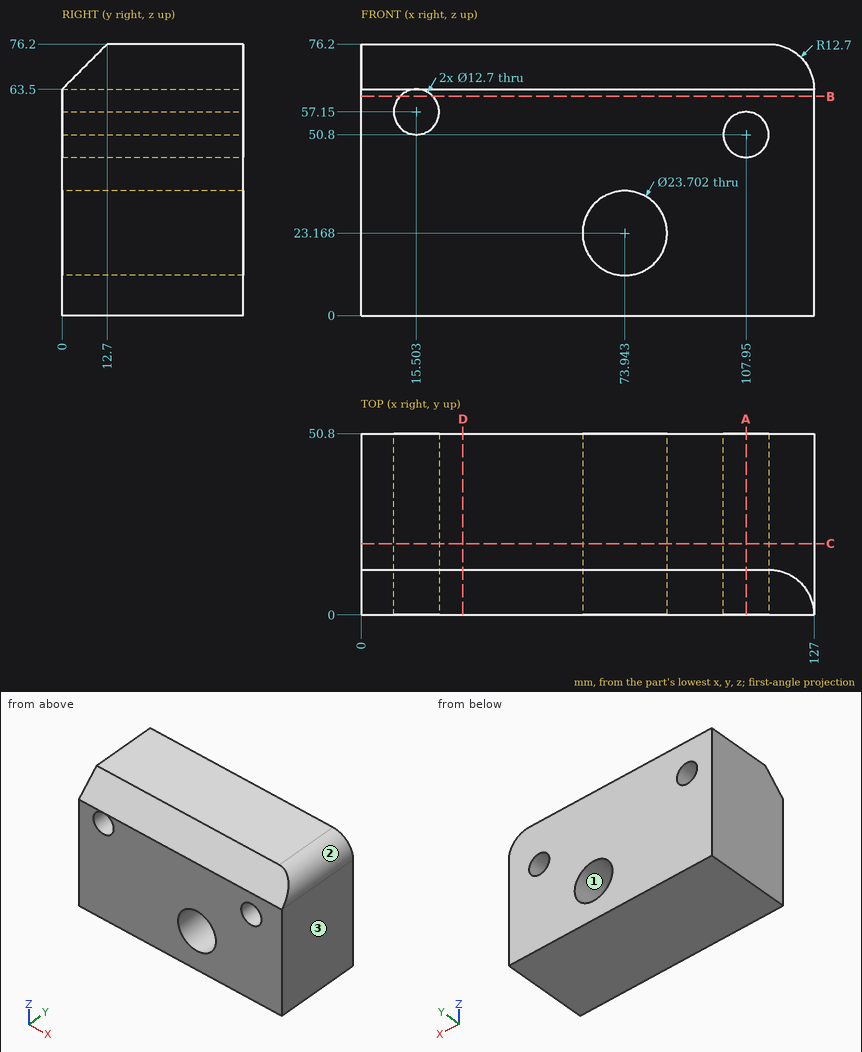
Part print with two shaded views. Sizes in mm from the minimum x, y, z corner. Coordinates: 2 decimals unless noted, no trailing zeros. Order: outer loops, then holes, each group sorted by start corner. A loop starts at its lowest first (then second) coordinate and runs counter-clockwise, first axis right, second up. Notation, with made-up numbers: M 65,30 L 82,30 A18 ccw 82,36 Z; hole C 10.25,18 d8. An arc over 180 degrees is marked long. Use a Markdown table: item, result.
(1) Cut at B-B on z = 61.5. Write the cut outline in (x, y).
A:
| item | result |
|---|---|
| outline | M 0,0 L 10.88,0 L 10.88,50.8 L 0,50.8 Z; M 20.13,0 L 127,0 L 127,50.8 L 20.13,50.8 Z |
(2) Probe L1, parallel to Z at x = 107.95, y = 18.5; L2, parallel to Z at x = 80.5, y = 31 (1 decimal); L3, parallel to X at y = 21.5, z = 20. List the from-to ranges inside material, lowest first.
A:
| item | result |
|---|---|
| L1 | z = 0 to 44.45, 57.15 to 76.2 |
| L2 | z = 0 to 13.3, 33 to 76.2 |
| L3 | x = 0 to 62.52, 85.36 to 127 |
(3) Cut at C-C on y = 20. State how many separate pieces and enclosed holes the cut face has, then the cut area to 3 significant figures.
A:
| item | result |
|---|---|
| separate pieces | 1 |
| enclosed holes | 3 |
| area | 8,950 mm^2 |
(4) Cut at D-D on x = 28.5. Write the cut outline in (y, z).
A:
| item | result |
|---|---|
| outline | M 0,0 L 50.8,0 L 50.8,76.2 L 12.7,76.2 L 0,63.5 Z |
(5) Cut at A-A on x = 107.95. Write the cut outline in (y, z).
A:
| item | result |
|---|---|
| outline | M 0,0 L 50.8,0 L 50.8,44.45 L 0,44.45 Z; M 0,57.15 L 50.8,57.15 L 50.8,76.2 L 12.7,76.2 L 0,63.5 Z |
(6) Pull direction Z, two halves, no side cores. Call the marked faces 1, 2 and 3: released by +Z, released by -Z, zero draft, split by the parting line, or undercut.
A:
| item | result |
|---|---|
| face 1 | undercut |
| face 2 | released by +Z |
| face 3 | zero draft |
